from build123d import *

# Parameters (mm, degrees)
SKETCH1_W               = 190.5
SKETCH1_H               = 190.5
BOSS_EXTRUDE1_DEPTH     = 12.7
FILLET1_R               = 7.62
BOSS_EXTRUDE3_START     = 19.05
BOSS_EXTRUDE3_DEPTH     = 19.05
CIRPATTERN1_COUNT       = 4
SKETCH8_R               = 6.223
CUT_EXTRUDE2_DEPTH      = 25.4
CUT_EXTRUDE6_DEPTH      = 137.044211564
CUT_EXTRUDE6_DEPTH_BACK = 137.044211564
SKETCH10_R              = 6.223
SKETCH11_R              = 6.35
SKETCH11_R_2            = 3.2385
CUT_EXTRUDE7_DEPTH      = 19.05
SKETCH11_4_R            = 3.2385
CUT_EXTRUDE8_DEPTH      = 139.395041457
FILLET3_R               = 12.7
BOSS_EXTRUDE5_DEPTH     = 12.7


with BuildPart() as part:
    # Sketch1 → Boss-Extrude1 (new body)
    with BuildSketch(Plane(origin=(0, 0, 0), x_dir=(1, 0, 0), z_dir=(0, 1, 0))):
        Rectangle(SKETCH1_W, SKETCH1_H)
    extrude(amount=BOSS_EXTRUDE1_DEPTH)

    # Fillet1
    fillet1_edges = [part.edges().sort_by_distance(p)[0] for p in [
        (95.25, 6.35, 95.25),
        (-95.25, 6.35, 95.25),
        (-95.25, 6.35, -95.25),
        (95.25, 6.35, -95.25),
    ]]
    fillet(fillet1_edges, radius=FILLET1_R)

    # Sketch7 → Boss-Extrude3 (add)
    with BuildSketch(Plane(origin=(0, 12.7, 0), x_dir=(1, 0, 0), z_dir=(0, 1, 0)).offset(BOSS_EXTRUDE3_START)):
        with BuildLine():
            Line((67.396822189, 67.396822189), (93.018153673, 93.018153673))
            ThreePointArc((93.018153673, 93.018153673), (90.546047755, 94.669962038), (87.63, 95.25))
            Line((87.63, 95.25), (62.921077964, 95.25))
            Line((62.921077964, 95.25), (49.265209936, 81.594131972))
            ThreePointArc((49.265209936, 81.594131972), (58.761367718, 75.045086089), (67.396822189, 67.396822189))
        make_face()
        with BuildLine():
            ThreePointArc((95.25, 87.63), (94.669962038, 90.546047755), (93.018153673, 93.018153673))
            Line((93.018153673, 93.018153673), (67.396822189, 67.396822189))
            ThreePointArc((67.396822189, 67.396822189), (75.045086089, 58.761367718), (81.594131972, 49.265209936))
            Line((81.594131972, 49.265209936), (95.25, 62.921077964))
            Line((95.25, 62.921077964), (95.25, 87.63))
        make_face()
    boss_extrude3 = extrude(amount=-BOSS_EXTRUDE3_DEPTH)

    # CirPattern1: Boss-Extrude3 ×4 about axis
    cirpattern1_axis = Axis((0, 0, 0), (0, 1, 0))
    for i in range(1, CIRPATTERN1_COUNT):
        add(boss_extrude3.rotate(cirpattern1_axis, i * 360 / CIRPATTERN1_COUNT))

    # Sketch8 → Cut-Extrude2 (cut)
    with BuildSketch(Plane(origin=(0, 12.7, 0), x_dir=(1, 0, 0), z_dir=(0, 1, 0))):
        with Locations(Location((0, 82.55, 0), (0, 0, 270))):
            Circle(SKETCH8_R)
        with Locations(Location((58.371664787, 58.371664787, 0), (0, 0, 270))):
            Circle(SKETCH8_R)
        with Locations(Location((82.55, 0, 0), (0, 0, 270))):
            Circle(SKETCH8_R)
        with Locations(Location((58.371664787, -58.371664787, 0), (0, 0, 270))):
            Circle(SKETCH8_R)
        with Locations(Location((0, -82.55, 0), (0, 0, 270))):
            Circle(SKETCH8_R)
        with Locations(Location((-58.371664787, -58.371664787, 0), (0, 0, 270))):
            Circle(SKETCH8_R)
        with Locations(Location((-82.55, 0, 0), (0, 0, 270))):
            Circle(SKETCH8_R)
        with Locations(Location((-58.371664787, 58.371664787, 0), (0, 0, 270))):
            Circle(SKETCH8_R)
    extrude(amount=-CUT_EXTRUDE2_DEPTH, mode=Mode.SUBTRACT)

    # Sketch10 → Cut-Extrude6 (cut, two sides: drawn at the far end of the back side and taken through both)
    with BuildSketch(Plane(origin=(0, 12.7, 0), x_dir=(1, 0, 0), z_dir=(0, 1, 0)).offset(-CUT_EXTRUDE6_DEPTH_BACK)):
        with BuildLine():
            Line((95.25, -62.921077964), (95.25, 38.1))
            Line((95.25, 38.1), (38.1, 38.1))
            Line((38.1, 38.1), (38.1, 95.25))
            Line((38.1, 95.25), (-62.921077964, 95.25))
            Line((-62.921077964, 95.25), (-49.265209936, 81.594131972))
            ThreePointArc((-49.265209936, 81.594131972), (-67.396822189, 67.396822189), (-81.594131972, 49.265209936))
            Line((-81.594131972, 49.265209936), (-95.25, 62.921077964))
            Line((-95.25, 62.921077964), (-95.25, -62.921077964))
            Line((-95.25, -62.921077964), (-81.594131972, -49.265209936))
            ThreePointArc((-81.594131972, -49.265209936), (-67.396822189, -67.396822189), (-49.265209936, -81.594131972))
            Line((-49.265209936, -81.594131972), (-62.921077964, -95.25))
            Line((-62.921077964, -95.25), (62.921077964, -95.25))
            Line((62.921077964, -95.25), (49.265209936, -81.594131972))
            ThreePointArc((49.265209936, -81.594131972), (67.396822189, -67.396822189), (81.594131972, -49.265209936))
            Line((81.594131972, -49.265209936), (95.25, -62.921077964))
        make_face()
        with Locations((-58.371664787, -58.371664787)):
            Circle(SKETCH10_R, mode=Mode.SUBTRACT)
        with Locations((-82.55, 0)):
            Circle(SKETCH10_R, mode=Mode.SUBTRACT)
        with Locations((0, -82.55)):
            Circle(SKETCH10_R, mode=Mode.SUBTRACT)
        with Locations((58.371664787, -58.371664787)):
            Circle(SKETCH10_R, mode=Mode.SUBTRACT)
        with Locations((-58.371664787, 58.371664787)):
            Circle(SKETCH10_R, mode=Mode.SUBTRACT)
        with Locations((0, 82.55)):
            Circle(SKETCH10_R, mode=Mode.SUBTRACT)
        with Locations((82.55, 0)):
            Circle(SKETCH10_R, mode=Mode.SUBTRACT)
    extrude(amount=CUT_EXTRUDE6_DEPTH + CUT_EXTRUDE6_DEPTH_BACK, mode=Mode.SUBTRACT)


with BuildPart() as cut_extrude6_kept_piece:
    # of the separate pieces the step leaves, the one the design keeps (cut_extrude6_pieces_kept)
    add(part.part.solids().sort_by_distance((38.1, 0, -38.1))[0])

    # Sketch11 → Cut-Extrude7 (cut)
    with BuildSketch(Plane(origin=(0, 31.75, 0), x_dir=(1, 0, 0), z_dir=(0, 1, 0))):
        with Locations(Location((82.55, 82.55, 0), (0, 0, 270))):
            Circle(SKETCH11_R)
        with Locations(Location((82.55, 82.55, 0), (0, 0, 270))):
            Circle(SKETCH11_R_2, mode=Mode.SUBTRACT)
    extrude(amount=-CUT_EXTRUDE7_DEPTH, mode=Mode.SUBTRACT)

    # Sketch11<4> → Cut-Extrude8 (cut, through all)
    with BuildSketch(Plane(origin=(0, 31.75, 0), x_dir=(1, 0, 0), z_dir=(0, 1, 0))):
        with Locations(Location((82.55, 82.55, 0), (0, 0, 270))):
            Circle(SKETCH11_4_R)
    extrude(amount=-CUT_EXTRUDE8_DEPTH, mode=Mode.SUBTRACT)

    # Fillet3
    fillet3_edges = [cut_extrude6_kept_piece.edges().sort_by_distance(p)[0] for p in [
        (38.1, 6.35, -95.25),
        (38.1, 6.35, -38.1),
        (95.25, 6.35, -38.1),
    ]]
    fillet(fillet3_edges, radius=FILLET3_R)

    # Sketch12 → Boss-Extrude5 (add)
    with BuildSketch(Plane(origin=(0, 12.7, 0), x_dir=(1, 0, 0), z_dir=(0, 1, 0))):
        with BuildLine():
            ThreePointArc((38.1, 82.55), (41.819743879, 91.530256121), (50.8, 95.25))
            Line((50.8, 95.25), (19.05, 95.25))
            Line((19.05, 95.25), (19.05, 64.77))
            Line((19.05, 64.77), (38.1, 64.77))
            Line((38.1, 64.77), (38.1, 82.55))
        make_face()
        with BuildLine():
            Line((82.55, 38.1), (64.77, 38.1))
            Line((64.77, 38.1), (64.77, 19.05))
            Line((64.77, 19.05), (95.25, 19.05))
            Line((95.25, 19.05), (95.25, 50.8))
            ThreePointArc((95.25, 50.8), (91.530256121, 41.819743879), (82.55, 38.1))
        make_face()
        with BuildLine():
            Line((38.1, 50.8), (38.1, 64.77))
            Line((38.1, 64.77), (19.05, 64.77))
            ThreePointArc((19.05, 64.77), (32.441077964, 32.441077964), (64.77, 19.05))
            Line((64.77, 19.05), (64.77, 38.1))
            Line((64.77, 38.1), (50.8, 38.1))
            ThreePointArc((50.8, 38.1), (41.819743879, 41.819743879), (38.1, 50.8))
        make_face()
    extrude(amount=-BOSS_EXTRUDE5_DEPTH)


solid = cut_extrude6_kept_piece.part
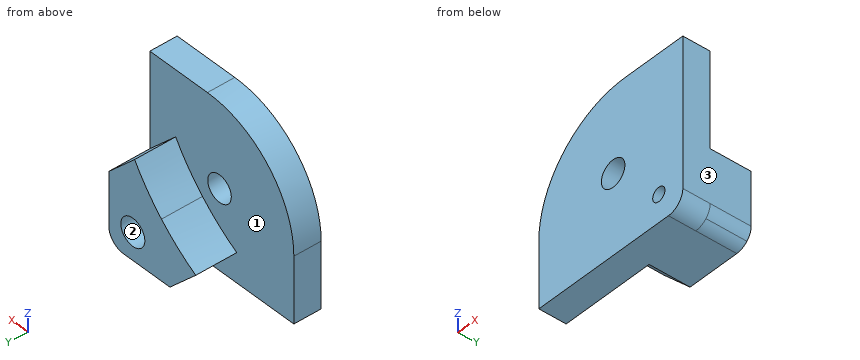
Design review of the part built by this model. Coordinates are the model's own, in mm. Face numbers are marked on the shaded views. Give positions to 0.01 mm unless a question says otherwise; leave off trailing zeros. Order: outer loops, then holes, each group sorted by start corner. A loop starts at its lowest first (then second) coordinate and runs counter-clockwise, first axis right, second up. Notation, with made-up numbers: (60.25, 42.25) - (80.25, 42.25) arc R24 ccw to (80.25, 53.25) - close; hole circle Ø1 at (1.25, 75). An arc over 180 degrees is marked (long way). Use CSV: the item, a comma, the result in double quotes. Start each with the question number.
Q1. Take a section at B-B (x = 82.55). State the section outline as (y, z) points, and give its area (3 significant figures).
Q2. Draft analysis for pull direction X (two halves, no side actions). For the marked faces 1, 2 and 3, state which applies: pulls with the +X half, pulls with the -X half, needs draft (parallel to the pull), parting line crosses it, or undercut.
Q3. For line 1 (Y direction, x = 79, z = -80); line 2 (Z direction, x = 57, y = 6); line 3 (Z direction, x = 79, y = 25), list the stretches that pass through material, from the lowest coordinate up.
Q4. For P1, Ø1.5, axis at x = 37.5, z = -36.5, coming from the +Y side; P2, Ø5, axis at x = 55, y = 27.5, coming from the +Z side; P3, Ø1.5, axis at x = 47.5, y = 15.5, coming from the +Z side; P4, Ø4, axis at y = 19, z = -49.5, coming from the +X side, all flat-tipped, find the tip position at first contact; note any pin that passes through.
Q5. Take a section at C-C (z = -61). State the section outline as (x, y) points, and give its area (3 significant figures).
Q6. Take a section at A-A (y = 18). State the section outline as (x, z) points, and give its area (3 significant figures).
Q7. Take a section at D-D (z = -82.55). State the section outline as (x, y) points, and give its area (3 significant figures).
Calculated:
1,outline,"(0, -95.25) - (31.75, -95.25) - (31.75, -88.9) - (12.7, -88.9) - (12.7, -85.79) - (0, -85.79) - close; (0, -79.31) - (12.7, -79.31) - (12.7, -76.2) - (31.75, -76.2) - (31.75, -50.22) - (12.7, -50.22) - (12.7, -19.05) - (0, -19.05) - close"
1,area,"1,500 mm²"
2,face 1,"needs draft"
2,face 2,"undercut"
2,face 3,"pulls with the +X half"
3,line 1,"y = 0 to 12.7"
3,line 2,"z = -95.25 to -64.44, -52.3 to -19.72"
3,line 3,"z = -95.25 to -87.81, -77.29 to -53.33"
4,P1,"stops at y = 12.7"
4,P2,"stops at z = -76.02"
4,P3,"passes through"
4,P4,"stops at x = 83.83"
5,outline,"(19.21, 0) - (52.73, 0) - (52.73, 12.7) - (19.21, 12.7) - close; (64.01, 0) - (95.25, 0) - (95.25, 12.7) - (93.33, 12.7) - (93.33, 31.75) - (73.24, 31.75) - (73.24, 12.7) - (64.01, 12.7) - close"
5,area,"1,210 mm²"
6,outline,"(49.27, -81.59) - (62.92, -95.25) - (87.63, -95.25) arc R7.62 ccw to (95.25, -87.63) - (95.25, -62.92) - (81.59, -49.27) arc R95.31 cw to start; hole circle Ø12.7 at (82.55, -82.55)"
6,area,"1,180 mm²"
7,outline,"(19.05, 0) - (79.31, 0) - (79.31, 12.7) - (76.2, 12.7) - (76.2, 31.75) - (50.22, 31.75) - (50.22, 12.7) - (19.05, 12.7) - close; (85.79, 0) - (95.25, 0) - (95.25, 31.75) - (88.9, 31.75) - (88.9, 12.7) - (85.79, 12.7) - close"
7,area,"1,500 mm²"
